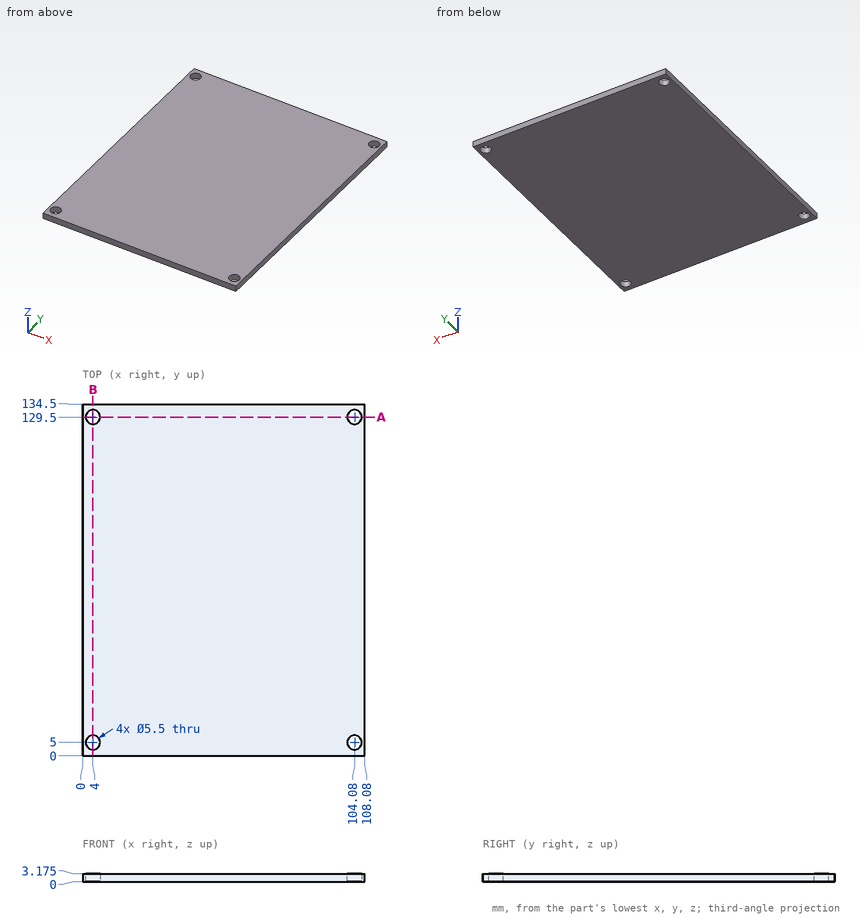
Input: dimensioned drawing with shaded views. Units: mm. Origin: part minimum x, y, z. Give positions to 0.01 mm unless a question says otherwise; leave off trailing zeros. Write each loop counter-clockwise with the first axis right and the second up, starting at its lowest first coordinate (ties: lowest second). Pieces come first, ordered by that corner, then holes. Notation, with made-up numbers: M 88,-4 L 118,-4 A11 ccw 118,16 Z; hole C 32,48 d1. An arc over 180 degrees is marked long. Return JSON: item names as keys, results as strings. Group by question number.
1) Cut plane B-B, the plane x = 4. Output: boundary loops of the cut face in (y, z) (3 decimals).
2) Material intervals for line 1 along X through (y, z) = (129.5, 2.55); line 2 along Y through (x, z) = (4, 1.15); line 3 along Y through (x, z) = (102, 2.5), sorted ascending. Write a range as [from, to].
3) Pin query (flat end, axial travel): P1, Ø3, axis at x = 49, y = 114, coming from the -Z side. Return the tip coordinate at first contact, or that it passes through.
4) Cut plane A-A, the plane y = 129.5. Give the number of separate pieces and of enclosed holes in the cut face, plus the area to 3 significant figures.
Recorded:
{
 "1": {"outline": "M 0,0 L 2.25,0 L 2.25,3.175 L 0,3.175 Z; M 7.75,0 L 126.75,0 L 126.75,3.175 L 7.75,3.175 Z; M 132.25,0 L 134.5,0 L 134.5,3.175 L 132.25,3.175 Z"},
 "2": {"line 1": "x = [0, 1.25], [6.75, 101.33], [106.83, 108.08]", "line 2": "y = [0, 2.25], [7.75, 126.75], [132.25, 134.5]", "line 3": "y = [0, 3.2], [6.8, 127.7], [131.3, 134.5]"},
 "3": {"P1": "stops at z = 0"},
 "4": {"separate pieces": "3", "enclosed holes": "0", "area": "308 mm²"}
}
